Build history of the part. All positions in model axes, mm. A direction names the side the tool comes from. Round coordinates to 2 decimals unless told otherwise and drop trailing zeros. Write each loop counter-clockwise with the first axis right and the second up, starting at its lowest first coordinate (ties: lowest second). Pieces come first, ordered by that corner, then holes.
Item 1: Band-saw the part on B-B, the plane z = 3. Write the cut outline in (x, y).
Item 2: 3-axis set-ups, long thin cutter, end or side, ignore diameter. For faces 4 (the flat face through (93, 11.43, 3)), 5 (the flat face through (91, 29, 0)): which of +Z, -Z, +X, -X, +Y, -Y reach the whole face in a straight line?
Item 3: Band-saw the part on C-C, the plane y = 19.5. Write the cut outline in (x, z).
Item 4: Mould opens along X. For faces 1 (the flat face through (0, 28, 3)), 2 (the flat face through (91, 21.59, 3)), 3 (the flat face through (91, 0, 3)) say: +X half, -X half, draft (parallel to the pull), parting line (faces both ways), or undercut.
Item 5: Band-saw the part on A-A, the plane x = 63.5. Write the cut outline in (y, z), then the cut area to 3 significant figures.
Item 6: Wall check: probe 1 along Y at (x, z) = (43, 5.75). Give the ranges that are in metal, low to high.
```python
from build123d import *

# Parameters (mm, degrees)
F0_W     = 184.15
F0_H     = 57.15
F1_DEPTH = 6.35


with BuildPart() as f1:
    # F0 (on Top) → F1 (new body)
    with BuildSketch(Plane.XY):
        with Locations((92.075, 28.575)):
            Rectangle(F0_W, F0_H)
        with BuildLine():
            Line((160.02, 11.43), (24.13, 11.43))
            ThreePointArc((24.13, 11.43), (20.537898, 12.917898), (19.05, 16.51))
            ThreePointArc((19.05, 16.51), (20.537898, 20.102102), (24.13, 21.59))
            Line((24.13, 21.59), (160.02, 21.59))
            ThreePointArc((160.02, 21.59), (163.612102, 20.102102), (165.1, 16.51))
            ThreePointArc((165.1, 16.51), (163.612102, 12.917898), (160.02, 11.43))
        make_face(mode=Mode.SUBTRACT)
    extrude(amount=F1_DEPTH)


solid = f1.part
```
Results:
1. outline: (0, 0) - (184.15, 0) - (184.15, 57.15) - (0, 57.15) - close; hole (19.05, 16.51) arc R5.08 ccw to (24.13, 11.43) - (160.02, 11.43) arc R5.08 ccw to (165.1, 16.51) arc R5.08 ccw to (160.02, 21.59) - (24.13, 21.59) arc R5.08 ccw to start
2. face 4: +Z, -Z
2. face 5: -Z, +X, -X, +Y, -Y
3. outline: (0, 0) - (20.02, 0) - (20.02, 6.35) - (0, 6.35) - close; (164.13, 0) - (184.15, 0) - (184.15, 6.35) - (164.13, 6.35) - close
4. face 1: -X half
4. face 2: undercut
4. face 3: draft
5. outline: (0, 0) - (11.43, 0) - (11.43, 6.35) - (0, 6.35) - close; (21.59, 0) - (57.15, 0) - (57.15, 6.35) - (21.59, 6.35) - close
5. area: 298 mm2
6. probe 1: y = 0 to 11.43, 21.59 to 57.15
